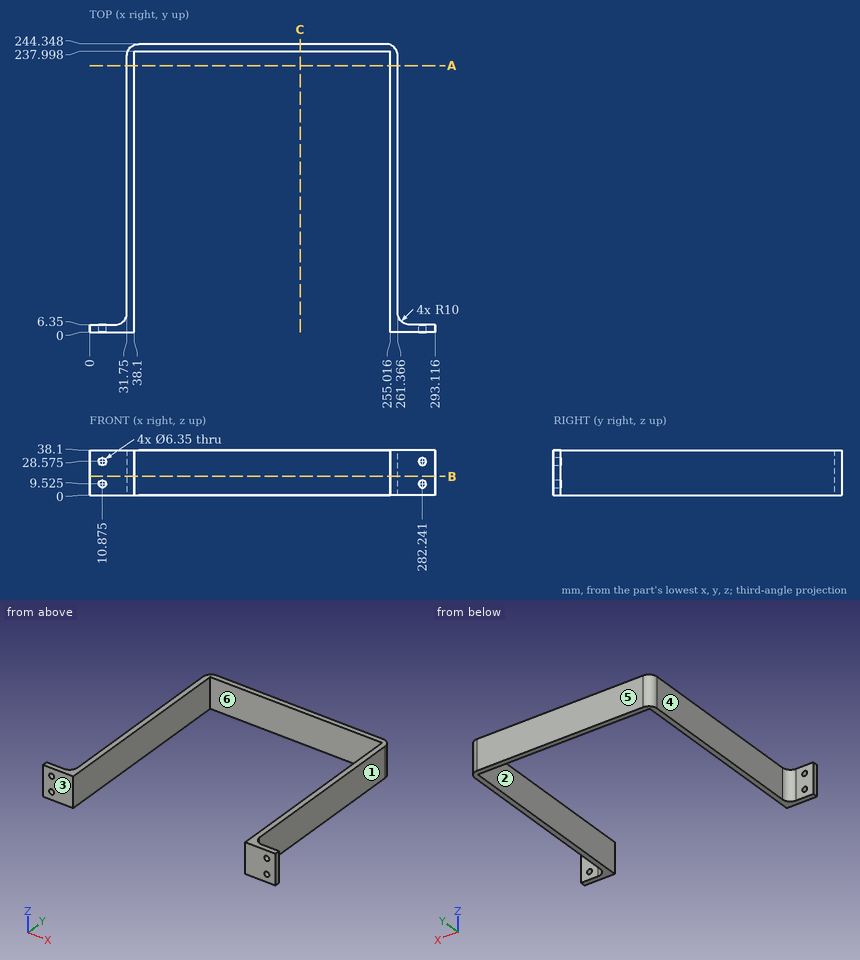
For this review, use the dimensioned drawing (mm, ordinates from the lowest corner) and the shaded views. A direction names the side the tool comes from. Coordinates: 2 decimals unless noted, no trailing zeros. Order: outer loops, then holes, each group sorted by start corner. A loop starts at its lowest first (then second) coordinate and runs counter-clockwise, first axis right, second up. Notation, with made-up numbers: (23, -31) - (66, -31) arc R20 ccw to (66, -20) - close; hole circle Ø6 at (-17.5, -20.5). An arc over 180 degrees is marked (long way). Answer in a Markdown table with one row per item.
(1) Consider section A-A on y = 226. State the section outline as (x, z) points, plus the area to 3 significant figures.
Checked values:
| item | result |
|---|---|
| outline | (31.75, 0) - (38.1, 0) - (38.1, 38.1) - (31.75, 38.1) - close; (255.02, 0) - (261.37, 0) - (261.37, 38.1) - (255.02, 38.1) - close |
| area | 484 mm^2 |
(2) Wall thickness on line 1 along X through (y, z) = (89, 31); line 2 along Y through (x, z) = (125.5, 18); line 3 along Y through (x, z) = (22.5, 18.5): over which ranges is each line inside the solid? List them lowest first. Write a range as from..to.
Checked values:
| item | result |
|---|---|
| line 1 | 31.75..38.1, 255.02..261.37 |
| line 2 | 238..244.35 |
| line 3 | 0..6.38 |
(3) The part is to be moulded in two halves that separate along X. For the marked faces 1, 2 and 3, say which applies: released by +X, released by -X, zero draft, split by the parting line, or undercut.
Checked values:
| item | result |
|---|---|
| face 1 | released by +X |
| face 2 | undercut |
| face 3 | zero draft |
(4) Clearance check with flat-ended pins moving along their axes: pin 1 (11 mm diameter, centred on x = 15, z = 10.5, fed in from +Y); pin 2 (12 mm diameter, centred on x = 83, z = 23.5, fed in from -Y); pin 3 (10 mm diameter, centred on y = 203.5, z = 19.5, fed in from -X). State where each tip first meets the part, or that it passes through.
Checked values:
| item | result |
|---|---|
| pin 1 | y = 6.35 |
| pin 2 | y = 238 |
| pin 3 | x = 31.75 |
(5) Consider section B-B on z = 16. State the section outline as (x, y) points, plus the area to 3 significant figures.
Checked values:
| item | result |
|---|---|
| outline | (0, 0) - (38.1, 0) - (38.1, 238) - (255.02, 238) - (255.02, 0) - (293.12, 0) - (293.12, 6.35) - (271.37, 6.35) arc R10 cw to (261.37, 16.35) - (261.37, 234.35) arc R10 ccw to (251.37, 244.35) - (41.75, 244.35) arc R10 ccw to (31.75, 234.35) - (31.75, 16.35) arc R10 cw to (21.75, 6.35) - (0, 6.35) - close |
| area | 4,880 mm^2 |
(6) For the marked faces 4, 5 and 6, list the 3-axis set-ups (+Z, -Z, +X, -X, +Y, -Y) from which the entire face can be reached by the end or side of a thin tool; tool diameter is ignored.
Checked values:
| item | result |
|---|---|
| face 4 | +Z, -Z, -X, +Y |
| face 5 | +Z, -Z, +X, -X, +Y |
| face 6 | +Z, -Z, -Y |
(7) Consider section C-C on x = 178.5. State the section outline as (y, z) points, plus the area to 3 significant figures.
Checked values:
| item | result |
|---|---|
| outline | (238, 0) - (244.35, 0) - (244.35, 38.1) - (238, 38.1) - close |
| area | 242 mm^2 |
